from build123d import *

# Parameters (mm, degrees)
BASE_FLANGE1_DEPTH      = 45
SKETCH5_R               = 4.5
SKETCH5_R_2             = 1.3
CUT_EXTRUDE1_DEPTH      = 10
CUT_EXTRUDE5_DEPTH      = 68.5
CUT_EXTRUDE5_DEPTH_BACK = 68.5
CUT_EXTRUDE6_DEPTH      = 67.821078603
CUT_EXTRUDE6_DEPTH_BACK = 67.821078603
SKETCH9_R               = 1.3
FILLET1_R               = 2
EDGE_FLANGE2_DEPTH      = 34.34
EDGE_FLANGE3_DEPTH      = 34.34
FILLET2_R               = 2


# Sheet-metal steps are written as plain solids
with BuildPart() as part:
    # Sketch1 → Base-Flange1 (new body)
    with BuildSketch(Plane.XY):
        with BuildLine():
            Line((-20.5, 45), (-20.5, 3.33))
            ThreePointArc((-20.5, 3.33), (-19.524665581, 0.975334419), (-17.17, 0))
            Line((-17.17, 0), (17.17, 0))
            ThreePointArc((17.17, 0), (19.524665581, 0.975334419), (20.5, 3.33))
            Line((20.5, 3.33), (20.5, 45))
            Line((20.5, 45), (22.5, 45))
            Line((22.5, 45), (22.5, 3.33))
            ThreePointArc((22.5, 3.33), (20.938879144, -0.438879144), (17.17, -2))
            Line((17.17, -2), (-17.17, -2))
            ThreePointArc((-17.17, -2), (-20.938879144, -0.438879144), (-22.5, 3.33))
            Line((-22.5, 3.33), (-22.5, 45))
            Line((-22.5, 45), (-20.5, 45))
        make_face()
    extrude(amount=BASE_FLANGE1_DEPTH)

    # Sketch5 → Cut-Extrude1 (cut)
    with BuildSketch(Plane(origin=(0, 0, 0), x_dir=(-1, 0, 0), z_dir=(0, 1, 0))):
        with Locations(Location((0, 13, 0), (0, 0, 90))):
            Circle(SKETCH5_R)
        with Locations(Location((0, 5, 0), (0, 0, 90))):
            Circle(SKETCH5_R_2)
        with Locations(Location((-5.656854249, 7.343145751, 0), (0, 0, 90))):
            Circle(SKETCH5_R_2)
        with Locations(Location((-8, 13, 0), (0, 0, 90))):
            Circle(SKETCH5_R_2)
        with Locations(Location((-5.656854249, 18.656854249, 0), (0, 0, 90))):
            Circle(SKETCH5_R_2)
        with Locations(Location((0, 21, 0), (0, 0, 90))):
            Circle(SKETCH5_R_2)
        with Locations(Location((5.656854249, 18.656854249, 0), (0, 0, 90))):
            Circle(SKETCH5_R_2)
        with Locations(Location((8, 13, 0), (0, 0, 90))):
            Circle(SKETCH5_R_2)
        with Locations(Location((5.656854249, 7.343145751, 0), (0, 0, 90))):
            Circle(SKETCH5_R_2)
    extrude(amount=-CUT_EXTRUDE1_DEPTH, mode=Mode.SUBTRACT)

    # Sketch8 → Cut-Extrude5 (cut, two sides: drawn at the far end of the back side and taken through both)
    with BuildSketch(Plane(origin=(0, 0, 0), x_dir=(0, 0, -1), z_dir=(1, 0, 0)).offset(-CUT_EXTRUDE5_DEPTH_BACK)):
        with BuildLine():
            Line((-44.490485194, 25.752155493), (-38.833630945, 31.409009742))
            Line((-38.833630945, 31.409009742), (-36.712310601, 29.287689399))
            ThreePointArc((-36.712310601, 29.287689399), (-29.287689399, 29.287689399), (-29.287689399, 36.712310601))
            Line((-29.287689399, 36.712310601), (-31.409009742, 38.833630945))
            Line((-31.409009742, 38.833630945), (-25.752155493, 44.490485194))
            Line((-25.752155493, 44.490485194), (0, 18.738329701))
            Line((0, 18.738329701), (0, 54.044936655))
            Line((0, 54.044936655), (-47.344215892, 54.044936655))
            Line((-47.344215892, 54.044936655), (-47.344215892, -7.96210432))
            Line((-47.344215892, -7.96210432), (-26, -7.96210432))
            Line((-26, -7.96210432), (-26, 7.261670299))
            Line((-26, 7.261670299), (-44.490485194, 25.752155493))
        make_face()
    extrude(amount=CUT_EXTRUDE5_DEPTH + CUT_EXTRUDE5_DEPTH_BACK, mode=Mode.SUBTRACT)

    # Sketch9 → Cut-Extrude6 (cut, two sides: drawn at the far end of the back side and taken through both)
    with BuildSketch(Plane(origin=(0, 0, 0), x_dir=(0, 0, -1), z_dir=(1, 0, 0)).offset(-CUT_EXTRUDE6_DEPTH_BACK)):
        with Locations((-38.656854249, 27.343145751)):
            Circle(SKETCH9_R)
        with Locations((-41, 33)):
            Circle(SKETCH9_R)
        with Locations((-38.656854249, 38.656854249)):
            Circle(SKETCH9_R)
        with Locations((-33, 41)):
            Circle(SKETCH9_R)
        with Locations((-27.343145751, 38.656854249)):
            Circle(SKETCH9_R)
        with Locations((-25, 33)):
            Circle(SKETCH9_R)
        with Locations((-27.343145751, 27.343145751)):
            Circle(SKETCH9_R)
        with Locations((-33, 25)):
            Circle(SKETCH9_R)
    extrude(amount=CUT_EXTRUDE6_DEPTH + CUT_EXTRUDE6_DEPTH_BACK, mode=Mode.SUBTRACT)

    # Fillet1
    fillet1_edges = [part.edges().sort_by_distance(p)[0] for p in [
        (21.5, 18.738329701, 0),
        (21.5, 44.490485194, 25.752155493),
        (21.5, 38.833630945, 31.409009742),
        (21.5, 31.409009742, 38.833630945),
        (21.5, 25.752155493, 44.490485194),
        (21.5, 7.261670299, 26),
        (-21.5, 18.738329701, 0),
        (-21.5, 44.490485194, 25.752155493),
        (-21.5, 38.833630945, 31.409009742),
        (-21.5, 31.409009742, 38.833630945),
        (-21.5, 25.752155493, 44.490485194),
        (-21.5, 7.261670299, 26),
    ]]
    fillet(fillet1_edges, radius=FILLET1_R)

    # Edge-Flange2 section (across the edge) → Edge-Flange2 (add)
    with BuildSketch(Plane(origin=(-17.17, 0, 29.33), x_dir=(0, 0, -1), z_dir=(1, 0, 0))):
        with BuildLine():
            Line((-2, 3.33), (-2, 8.5))
            Line((-2, 8.5), (0, 8.5))
            Line((0, 8.5), (0, 3.33))
            ThreePointArc((0, 3.33), (0.975334419, 0.975334419), (3.33, 0))
            Line((3.33, 0), (3.33, -2))
            ThreePointArc((3.33, -2), (-0.438879144, -0.438879144), (-2, 3.33))
        make_face()
    extrude(amount=EDGE_FLANGE2_DEPTH)

    # Edge-Flange3 section (across the edge) → Edge-Flange3 (add)
    with BuildSketch(Plane(origin=(17.17, 0, -3.33), x_dir=(0, 0, 1), z_dir=(-1, 0, 0))):
        with BuildLine():
            Line((-2, 3.33), (-2, 8.5))
            Line((-2, 8.5), (0, 8.5))
            Line((0, 8.5), (0, 3.33))
            ThreePointArc((0, 3.33), (0.975334419, 0.975334419), (3.33, 0))
            Line((3.33, 0), (3.33, -2))
            ThreePointArc((3.33, -2), (-0.438879144, -0.438879144), (-2, 3.33))
        make_face()
    extrude(amount=EDGE_FLANGE3_DEPTH)

    # Fillet2
    fillet2_edges = [part.edges().sort_by_distance(p)[0] for p in [
        (-17.17, 8.5, 30.33),
        (17.17, 8.5, 30.33),
        (17.17, 8.5, -4.33),
        (-17.17, 8.5, -4.33),
    ]]
    fillet(fillet2_edges, radius=FILLET2_R)


solid = part.part
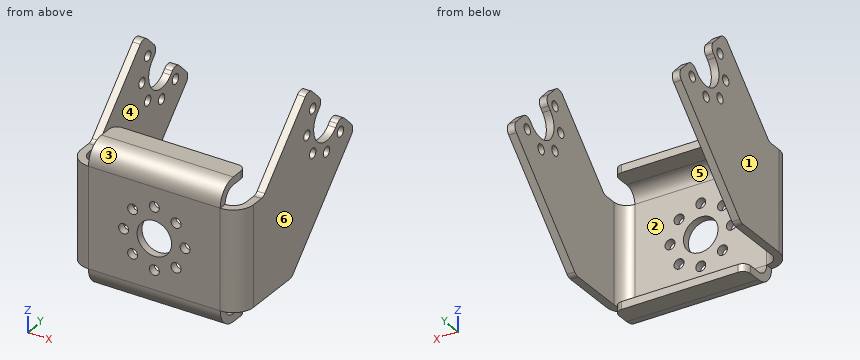
Read the model definition and answer for the solid it produces. Units are mm, in the model's axes. Face numbers are marked on the shaded views. A direction names the side the tool comes from. Coordinates: 2 decimals unless noted, no trailing zeros. Order: outer loops, then holes, each group sorted by start corner. A loop starts at its lowest first (then second) coordinate and runs counter-clockwise, first axis right, second up. Notation, with made-up numbers: (46.25, 17.25) - (70.25, 17.25) arc R25 ccw to (70.25, 53.25) - close; hole circle Ø6 at (0.5, 57). An arc over 180 degrees is marked (long way). Use one line per item in the form item = value.
(1) Given pin 1 Ø3 at (y, z) = (33, 25) entering from +X; pin 2 Ø3 at (x, z) = (8, 13) entering from +Y; pin 3 Ø1.6 at (y, z) = (3.5, -3) entering from -X; pin 4 Ø6 at (x, z) = (17.5, 31) entering from -Y, each flat-ended and moving along its own axis, determine where each tip first touches the part or whether it passes through.
Computed values:
pin_1 = 22.5
pin_2 = 0
pin_3 = -17.17
pin_4 = -1.6
(2) Straight lines are drawn through the part: L1, parallel to X at y = 17.5, z = 5; L2, parallel to Z at x = 7.5, y = 3; L3, parallel to Y at x = -2, z = 3.5. For each, find the intervals that lie inside material, in ascending order.
Computed values:
L1 = -22.5 to -20.5, 20.5 to 22.5
L2 = -5.32 to -3.31, 29.31 to 31.32
L3 = -2 to 0
(3) Section A-A, the plane x = 8 is taken. Give the vertices of the cut face in (y, z).
Computed values:
outline = (-2, 0) arc R5.33 ccw to (3.33, -5.33) - (8.5, -5.33) - (8.5, -3.33) - (3.33, -3.33) arc R3.33 cw to (0, 0) - (0, 11.7) - (-2, 11.7) - close; (-2, 14.3) - (0, 14.3) - (0, 26) arc R3.33 cw to (3.33, 29.33) - (8.5, 29.33) - (8.5, 31.33) - (3.33, 31.33) arc R5.33 ccw to (-2, 26) - close
(4) Section B-B, the plane y = 25 is taken. Give the vertices of the cut face in (x, z).
Computed values:
outline = (-22.5, 6.26) - (-20.5, 6.26) - (-20.5, 31.7) - (-22.5, 31.7) - close; (-22.5, 34.3) - (-20.5, 34.3) - (-20.5, 43.52) - (-22.5, 43.52) - close; (20.5, 6.26) - (22.5, 6.26) - (22.5, 31.7) - (20.5, 31.7) - close; (20.5, 34.3) - (22.5, 34.3) - (22.5, 43.52) - (20.5, 43.52) - close
(5) Section D-D, the plane z = 5 is taken. Give the vertices of the cut face in (x, y), then the cut area to 3 significant figures.
Computed values:
outline = (-22.5, 3.33) arc R5.33 ccw to (-17.17, -2) - (-1.3, -2) - (-1.3, 0) - (-17.17, 0) arc R3.33 cw to (-20.5, 3.33) - (-20.5, 23.74) - (-22.5, 23.74) - close; (1.3, -2) - (17.17, -2) arc R5.33 ccw to (22.5, 3.33) - (22.5, 23.74) - (20.5, 23.74) - (20.5, 3.33) arc R3.33 cw to (17.17, 0) - (1.3, 0) - close
area = 172 mm²
(6) For a pull along Z with two mould halves and no side action, classify the marked faces 1, 2 and 3 as pulls with the +Z half, pulls with the -Z half, needs draft (parallel to the pull), parting line crosses it, or undercut.
Computed values:
face_1 = needs draft
face_2 = undercut
face_3 = pulls with the +Z half
(7) Section C-C, the plane z = 13 is taken. Give the vertices of the cut face in (x, y), then the cut area to 3 significant figures.
Computed values:
outline = (-22.5, 3.33) arc R5.33 ccw to (-17.17, -2) - (-9.3, -2) - (-9.3, 0) - (-17.17, 0) arc R3.33 cw to (-20.5, 3.33) - (-20.5, 31.74) - (-22.5, 31.74) - close; (-6.7, -2) - (-4.5, -2) - (-4.5, 0) - (-6.7, 0) - close; (4.5, -2) - (6.7, -2) - (6.7, 0) - (4.5, 0) - close; (9.3, -2) - (17.17, -2) arc R5.33 ccw to (22.5, 3.33) - (22.5, 31.74) - (20.5, 31.74) - (20.5, 3.33) arc R3.33 cw to (17.17, 0) - (9.3, 0) - close
area = 181 mm²
(8) Which of the six approach directions +Z, -Z, +X, -X, +Y, -Y give full straight-line access (tool end or side, diameter ignored) to the marked faces 4, 5 and 6?
Computed values:
face_4 = +Z, -Z, +Y
face_5 = +X, -X, +Y
face_6 = +Z, -Z, +X, +Y, -Y
